Here's the drawing with two shaded views (mm, measured from the low corner). I have some questions. A direction names the side the tool comes from. Round coordinates to 2 decimals unless told otherwise and drop trailing zeros. Write each loop counter-clockwise with the first axis right and the second up, starting at its lowest first coordinate (ties: lowest second). Pieces come first, ordered by that corner, then holes. Notation, with made-up numbers: M 6,49 L 61,49 A13 ccw 61,60 Z; hole C 58.5,-28 d5. An arc over 180 degrees is marked long. Write item = value, one per line. Start each with the question number.
(1) I want a section at B-B (y = 60). List the corners of the cut face in (x, z) for me, and give its area (3 significant figures).
(2) I want a section at D-D (z = 26). List the corners of the cut face in (x, y) for me, and give its area (3 significant figures).
(3) I want a section at C-C (x = 142.5). List the corners of the cut face in (y, z) for me.
(4) I want a section at A-A (y = 80). List the corners of the cut face in (x, z) for me, and give its area (3 significant figures).
(5) Will these pins go through, and if not, where does the flat tip stop? pin 1 Ø10 at (x, z) = (30.5, 9.5) entering from -Y; pin 2 Ø8 at (y, z) = (111, 20.5) entering from +X (1 decimal); pin 3 Ø2 at (y, z) = (49, 10) entering from +X; pin 4 Ø16 at (x, y) = (111.25, 25.87) entering from -Z.
(6) If we mould it in two halves opening along X, with no side actions, what happens to the marked faces 1, 2 and 3? For each: released by +X, released by -X, zero draft, split by the parting line, or undercut.
(7) I need wall thicknesses on line 1 along Y through (x, z) = (51, 5) (1 decimal); line 2 along Y through (x, z) = (48.75, 7.5) (1 decimal); line 3 along Y through (x, z) = (80, 8). Which ranges of each line are inside material? Lowest first, please.
(8) On a 3-axis mill with a long thin cutter (end or side, diameter ignored), from which of +Z, -Z, +X, -X, +Y, -Y can I reach the whole of each face in a straight line? I mean the marked faces 4 and 5. Say none if no direction works.
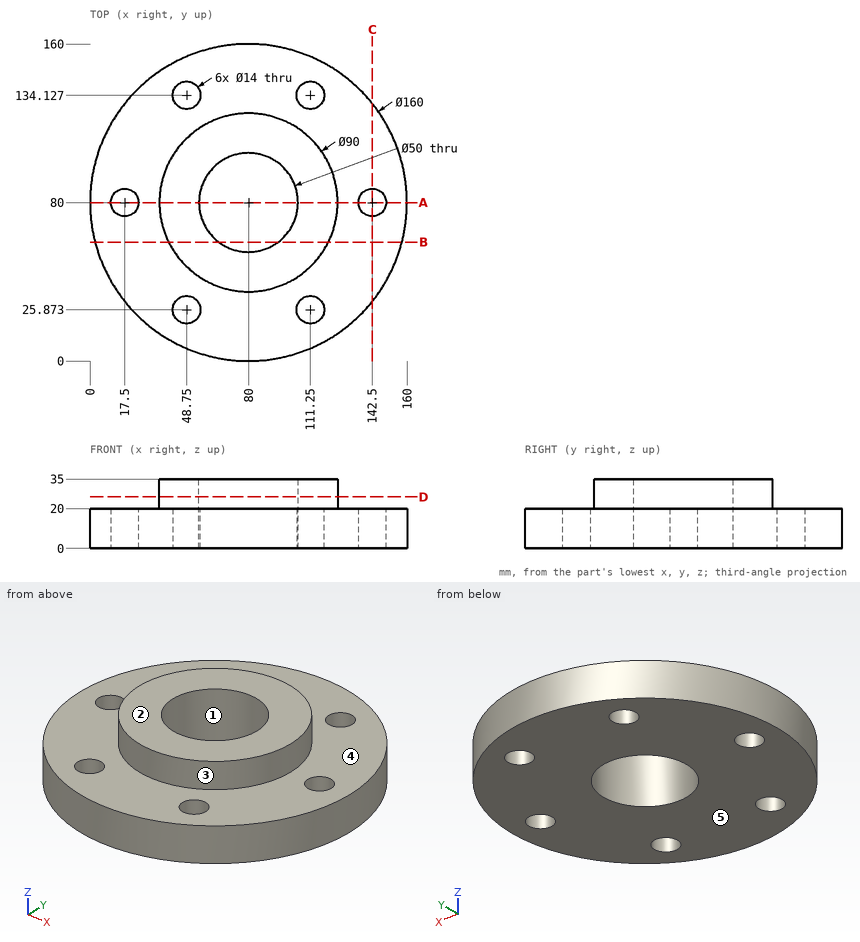
Returned:
q1.outline = M 2.54,0 L 65,0 L 65,35 L 39.69,35 L 39.69,20 L 2.54,20 Z; M 95,0 L 157.46,0 L 157.46,20 L 120.31,20 L 120.31,35 L 95,35 Z
q1.area = 3,260 mm²
q2.outline = C 80,80 d90; hole C 80,80 d50
q2.area = 4,400 mm²
q3.outline = M 30.06,0 L 73,0 L 73,20 L 30.06,20 Z; M 87,0 L 129.94,0 L 129.94,20 L 87,20 Z
q4.outline = M 0,0 L 10.5,0 L 10.5,20 L 0,20 Z; M 24.5,0 L 55,0 L 55,35 L 35,35 L 35,20 L 24.5,20 Z; M 105,0 L 135.5,0 L 135.5,20 L 125,20 L 125,35 L 105,35 Z; M 149.5,0 L 160,0 L 160,20 L 149.5,20 Z
q4.area = 2,240 mm²
q5.pin_1 = 13.52
q5.pin_2 = 155.3
q5.pin_3 = 154.16
q5.pin_4 = 0
q6.face_1 = undercut
q6.face_2 = zero draft
q6.face_3 = split by the parting line
q7.line_1 = 5.4 to 19.2, 32.5 to 127.5, 140.8 to 154.6
q7.line_2 = 6.4 to 18.9, 32.9 to 127.1, 141.1 to 153.6
q7.line_3 = 0 to 55, 105 to 160
q8.face_4 = +Z
q8.face_5 = -Z, +X, -X, +Y, -Y
